```python
from build123d import *

# Parameters (mm, degrees)
SKETCH1_R           = 55
SKETCH1_R_2         = 36
BOSS_EXTRUDE1_DEPTH = 12
SKETCH2_R           = 1.7
CUT_EXTRUDE1_DEPTH  = 79.70196948
SKETCH3_R           = 2.5
CUT_EXTRUDE2_DEPTH  = 5
CIRPATTERN1_COUNT   = 8


with BuildPart() as part:
    # Sketch1 → Boss-Extrude1 (new body)
    with BuildSketch(Plane(origin=(0, 0, 0), x_dir=(1, 0, 0), z_dir=(0, 1, 0))):
        with Locations(Location((0, 0, 0), (0, 0, 270))):
            Circle(SKETCH1_R)
        with Locations(Location((0, 0, 0), (0, 0, 270))):
            Circle(SKETCH1_R_2, mode=Mode.SUBTRACT)
    extrude(amount=BOSS_EXTRUDE1_DEPTH)

    # Sketch2 → Cut-Extrude1 (cut, symmetric)
    with BuildSketch(Plane(origin=(0, 12, 0), x_dir=(1, 0, 0), z_dir=(0, 1, 0))):
        with Locations(Location((45, 0, 0), (0, 0, 270))):
            Circle(SKETCH2_R)
    cut_extrude1 = extrude(amount=CUT_EXTRUDE1_DEPTH, both=True, mode=Mode.SUBTRACT)

    # Sketch3 → Cut-Extrude2 (cut)
    with BuildSketch(Plane(origin=(0, 12, 0), x_dir=(1, 0, 0), z_dir=(0, 1, 0))):
        with Locations(Location((45, 0, 0), (0, 0, 270))):
            Circle(SKETCH3_R)
    cut_extrude2 = extrude(amount=-CUT_EXTRUDE2_DEPTH, mode=Mode.SUBTRACT)

    # CirPattern1: Cut-Extrude1, Cut-Extrude2 ×8 about axis
    cirpattern1_axis = Axis((0, 0, 0), (0, 1, 0))
    add([cut_extrude1.rotate(cirpattern1_axis, i * 360 / CIRPATTERN1_COUNT) for i in range(1, CIRPATTERN1_COUNT)], mode=Mode.SUBTRACT)
    add([cut_extrude2.rotate(cirpattern1_axis, i * 360 / CIRPATTERN1_COUNT) for i in range(1, CIRPATTERN1_COUNT)], mode=Mode.SUBTRACT)


solid = part.part
```
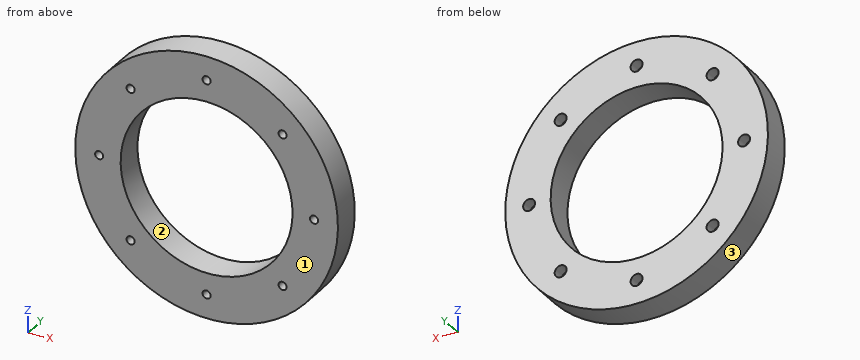
Design review of the part built by this model. Coordinates are the model's own, in mm. Face numbers are marked on the shaded views. Round coordinates to 2 decimals unless told otherwise and drop trailing zeros. Order: outer loops, then holes, each group sorted by start corner. A loop starts at its lowest first (then second) coordinate and runs counter-clockwise, first axis right, second up. Notation, with made-up numbers: M 47,28 L 86,28 A18 cw 86,59 Z; hole C 26.5,30 d7. An arc over 180 degrees is marked long. Put each result on its own line as item: value.
Q1. Insertion check: pin 1 Ø1 at (x, y) = (36, 4) entering from +Z; pin 2 Ø4 at (x, z) = (-45, 0) entering from +Y; pin 3 Ø5 at (y, z) = (8, 0) entering from -X. Each pin has a flat end and moves straight along its axis. Give the tip position at first contact, or say it passes through.
Reported:
pin 1: z = 42.01
pin 2: y = 7
pin 3: x = -55
Q2. Consider section B-B (z = 0). State the section outline as (x, y) points, and give its area (3 significant figures).
Reported:
outline: M -55,0 L -46.7,0 L -46.7,7 L -47.5,7 L -47.5,12 L -55,12 Z; M -43.3,0 L -36,0 L -36,12 L -42.5,12 L -42.5,7 L -43.3,7 Z; M 36,0 L 43.3,0 L 43.3,7 L 42.5,7 L 42.5,12 L 36,12 Z; M 46.7,0 L 55,0 L 55,12 L 47.5,12 L 47.5,7 L 46.7,7 Z
area: 358 mm²
Q3. Consider section A-A (x = 0). State the section outline as (y, z) points.
Reported:
outline: M 0,-55 L 12,-55 L 12,-47.5 L 7,-47.5 L 7,-46.7 L 0,-46.7 Z; M 0,-43.3 L 7,-43.3 L 7,-42.5 L 12,-42.5 L 12,-36 L 0,-36 Z; M 0,36 L 12,36 L 12,42.5 L 7,42.5 L 7,43.3 L 0,43.3 Z; M 0,46.7 L 7,46.7 L 7,47.5 L 12,47.5 L 12,55 L 0,55 Z
Q4. Consider section C-C (y = 4.75). State how many separate pieces and enclosed holes the cut face has, and give its area (3 significant figures).
Reported:
separate pieces: 1
enclosed holes: 9
area: 5,360 mm²
Q5. Draft analysis for pull direction X (two halves, no side actions). For the marked faces 1, 2 and 3, state which applies: released by +X, released by -X, zero draft, split by the parting line, or undercut.
Reported:
face 1: zero draft
face 2: undercut
face 3: split by the parting line
Q6. Consider section D-D (x = 22.5). State the section outline as (y, z) points.
Reported:
outline: M 0,-50.19 L 12,-50.19 L 12,-28.1 L 0,-28.1 Z; M 0,28.1 L 12,28.1 L 12,50.19 L 0,50.19 Z
Q7. To check wall thickness, follow line 1 (X direction, y = 2.25, z = 0); line 2 (Z direction, x = 8.5, y = 7.25); line 3 (X direction, y = 9, z = 45.5). State the ranges of each line that lie inside material, in increasing order.
Reported:
line 1: -55 to -46.7, -43.3 to -36, 36 to 43.3, 46.7 to 55
line 2: -54.34 to -34.98, 34.98 to 54.34
line 3: -30.9 to -2.45, 2.45 to 30.9
